Here's how the part is built. I have some questions about the finished solid (model axes, mm). Face numbers are marked on the shaded views. A direction names the side the tool comes from. Give positions to 0.01 mm unless a question says otherwise; leave off trailing zeros. Write each loop counter-clockwise with the first axis right and the second up, starting at its lowest first coordinate (ties: lowest second). Pieces come first, ordered by that corner, then holes. Notation, with made-up numbers: (42, 4.5) -> (61, 4.5) arc R22 ccw to (61, 13.5) -> close; hole circle Ø9 at (38.5, 83). An arc over 180 degrees is marked (long way). Put each result on its own line as item: value. Start each with the question number.
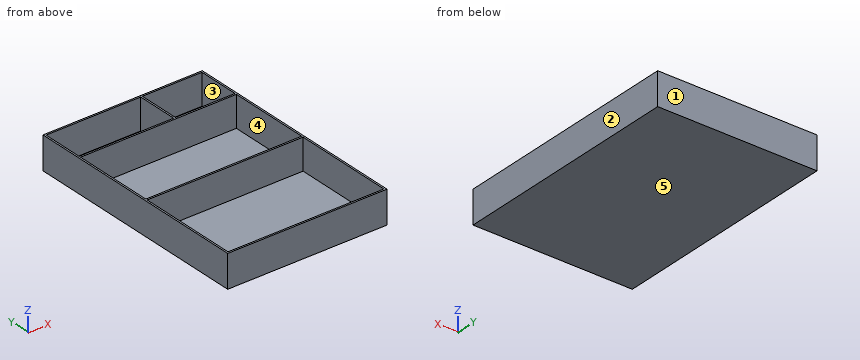
from build123d import *

# Parameters (mm, degrees)
SKETCH1_W           = 230.223051784
SKETCH1_H           = 338.919319135
BOSS_EXTRUDE1_DEPTH = 45.72
SHELL1_T            = 2.54
BOSS_EXTRUDE2_DEPTH = 45.72


with BuildPart() as part:
    # Sketch1 → Boss-Extrude1 (new body)
    with BuildSketch(Plane.XY):
        with Locations((20.509326923, 46.836837465)):
            Rectangle(SKETCH1_W, SKETCH1_H)
    extrude(amount=BOSS_EXTRUDE1_DEPTH)

    # Shell1
    shell1_openings = [part.faces().sort_by_distance(p)[0] for p in [
        (20.509326923, 46.836837464, 45.72),
    ]]
    offset(amount=SHELL1_T, openings=shell1_openings, kind=Kind.INTERSECTION)

    # Sketch2 → Boss-Extrude2 (add)
    with BuildSketch(Plane.XY):
        Polygon((45.097801031, 154.743483449), (-94.602198969, 154.743483449), (-94.602198969, 152.203483449), (-84.918790084, 152.203483449), (135.620852815, 152.203483449), (135.620852815, 154.743483449), (47.637801031, 154.743483449), (47.637801031, 216.296497032), (45.097801031, 216.296497032), align=None)
        Polygon((-94.602198969, 29.235642098), (-94.602198969, 30.557556356), (135.620852815, 30.557556356), (135.620852815, 27.965642098), (-94.602198969, 27.965642098), align=None)
    extrude(amount=BOSS_EXTRUDE2_DEPTH)


solid = part.part
1) I'm going to push a flat-ended pin straight in: pin 1 Ø4 at (x, y) = (17, 105) entering from +Z. Where does the tip first touch, or does it pass through?
2) I need wall thicknesses on probe 1 along Y at (x, z) = (-1.5, 19); probe 2 along X at (y, z) = (186.5, 1); probe 3 along X at (y, z) = (-65.5, 13.5). Which ranges of each line are inside material? Lowest first, please.
3) I want a section at B-B, the plane y = 187. Write out the boundary of the cut face in (x, z), and give its area (3 significant figures).
4) I want a section at D-D, the plane y = -29. Write out the boundary of the cut face in (x, z), and give its area (3 significant figures).
5) I want a section at C-C, the plane z = 18. Write out the boundary of the cut face in (x, y).
6) Which directions (+Z, -Z, +X, -X, +Y, -Y) give clear straight access to the entire face, cutting with the end or side of a thin tool? Please do the marked faces 4 and 5.
7) Thinking about a two-plate mould opening in Y: for the marked faces 1, 2 and 3, which applies, released by +Y, released by -Y, zero draft, split by the parting line, or undercut?
8) I want a section at A-A, the plane x = -39. Write out the boundary of the cut face in (y, z).
Established:
1. pin 1: stops at z = 0
2. probe 1: y = -125.16 to -122.62, 27.97 to 30.56, 152.2 to 154.74, 216.3 to 218.84
2. probe 2: x = -97.14 to -94.6, 45.1 to 47.64, 135.62 to 138.16
2. probe 3: x = -97.14 to -94.6, 135.62 to 138.16
3. outline: (-97.14, -2.54) -> (138.16, -2.54) -> (138.16, 45.72) -> (135.62, 45.72) -> (135.62, 0) -> (47.64, 0) -> (47.64, 45.72) -> (45.1, 45.72) -> (45.1, 0) -> (-94.6, 0) -> (-94.6, 45.72) -> (-97.14, 45.72) -> close
3. area: 946 mm2
4. outline: (-97.14, -2.54) -> (138.16, -2.54) -> (138.16, 45.72) -> (135.62, 45.72) -> (135.62, 0) -> (-94.6, 0) -> (-94.6, 45.72) -> (-97.14, 45.72) -> close
4. area: 830 mm2
5. outline: (-97.14, -125.16) -> (138.16, -125.16) -> (138.16, 218.84) -> (-97.14, 218.84) -> close; hole (-94.6, -122.62) -> (135.62, -122.62) -> (135.62, 27.97) -> (-94.6, 27.97) -> close; hole (-94.6, 30.56) -> (135.62, 30.56) -> (135.62, 152.2) -> (-94.6, 152.2) -> close; hole (-94.6, 154.74) -> (45.1, 154.74) -> (45.1, 216.3) -> (-94.6, 216.3) -> close; hole (47.64, 154.74) -> (135.62, 154.74) -> (135.62, 216.3) -> (47.64, 216.3) -> close
6. face 4: +Z
6. face 5: -Z, +X, -X, +Y, -Y
7. face 1: released by +Y
7. face 2: zero draft
7. face 3: undercut
8. outline: (-125.16, -2.54) -> (218.84, -2.54) -> (218.84, 45.72) -> (216.3, 45.72) -> (216.3, 0) -> (154.74, 0) -> (154.74, 45.72) -> (152.2, 45.72) -> (152.2, 0) -> (30.56, 0) -> (30.56, 45.72) -> (27.97, 45.72) -> (27.97, 0) -> (-122.62, 0) -> (-122.62, 45.72) -> (-125.16, 45.72) -> close
